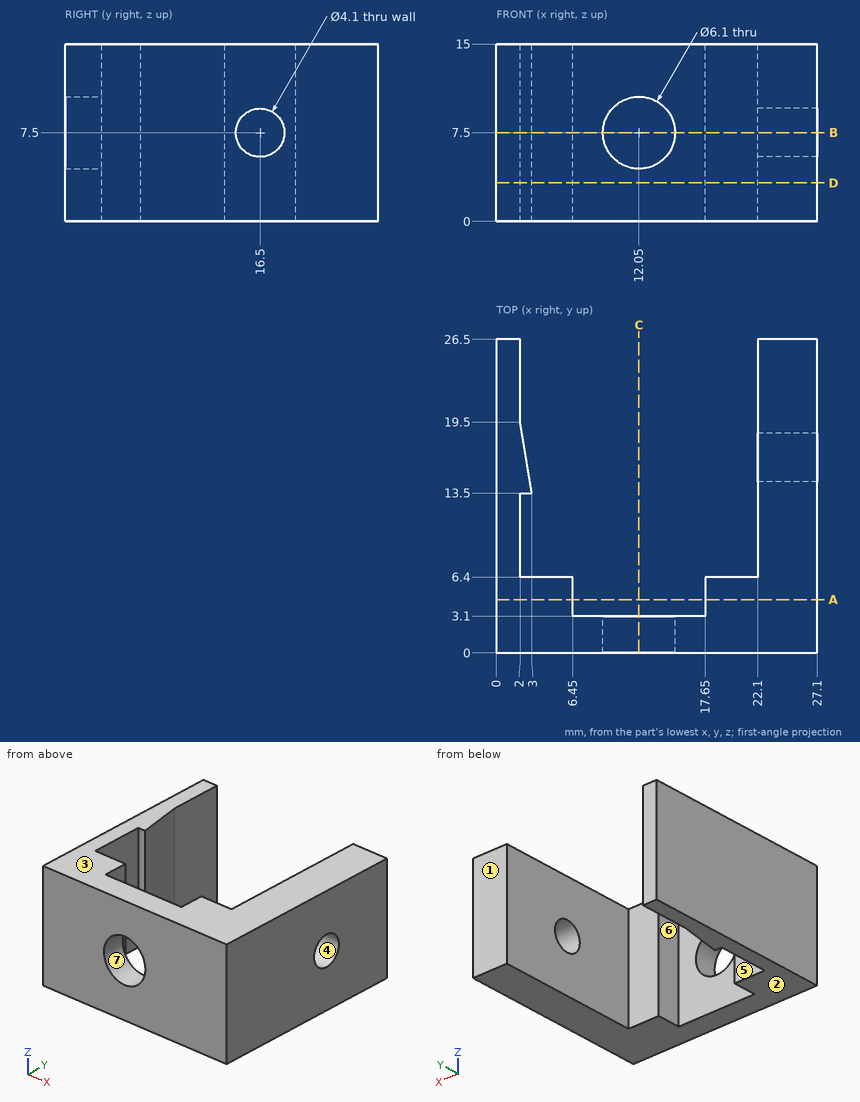
Verification items for this drawing (mm, ordinates from the low corner). A direction names the side the tool comes from. Coordinates: 2 decimals unless noted, no trailing zeros. Write each loop counter-clockwise with the first axis right and the second up, starting at its lowest first coordinate (ties: lowest second). Pieces come first, ordered by that corner, then holes. Notation, with made-up numbers: (76, 13.25) -> (100, 13.25) arc R9 cw to (100, 20.25) -> close; hole circle Ø2 at (-16.75, -34.5). An arc over 180 degrees is marked (long way). Use CSV: the item, a comma, the result in double quotes. Start each with the question number.
Item 1: Cross-section at C-C, the plane x = 12.05. Record the cut outline in (y, z).
Item 2: Thickness scan on line 1 (X direction, y = 25.25, z = 11.75); line 2 (Z direction, x = 23.1, y = 16.5); line 3 (X direction, y = 4.25, z = 9.25). Record the ranges inside material, lowest first.
Item 3: Cross-section at A-A, the plane y = 4.5. Record the cut outline in (x, z), plus the area to 4 significant figures.
Item 4: Depth check by flat-ended pin: pin 1 Ø1.3 at (x, z) = (20, 5.5) entering from +Y; pin 2 Ø1.7 at (y, z) = (5.5, 9) entering from -X; pin 3 Ø9 at (x, z) = (11, 10) entering from +Y. Enter the tip coordinate at first touch or a pass-through.
Item 5: Cross-section at D-D, the plane z = 3.25. Record the cut outline in (x, y), plus the area to 3 significant figures.
Item 6: Cross-section at B-B, the plane z = 7.5. Record the cut outline in (x, y).
Item 7: Set-up check for the marked faces 5, 6 and 7: record each of +Z, -Z, +X, -X, +Y, -Y from which the full face is reachable in a straight line by a thin tool's end or side.
Item 8: Mould release check, pull along Z, two halves, no side actions. Record for the marked faces 1, 2, 3 and 4: released by +Z, released by -Z, zero draft, split by the parting line, or undercut.
Answers:
1,outline,"(0, 0) -> (3.1, 0) -> (3.1, 4.45) -> (0, 4.45) -> close; (0, 10.55) -> (3.1, 10.55) -> (3.1, 15) -> (0, 15) -> close"
2,line 1,"0 to 2, 22.1 to 27.1"
2,line 2,"0 to 5.45, 9.55 to 15"
2,line 3,"0 to 6.45, 17.65 to 27.1"
3,outline,"(0, 0) -> (6.45, 0) -> (6.45, 15) -> (0, 15) -> close; (17.65, 0) -> (27.1, 0) -> (27.1, 15) -> (17.65, 15) -> close"
3,area,"238.5 mm^2"
4,pin 1,"y = 6.4"
4,pin 2,"x = 0"
4,pin 3,"y = 3.1"
5,outline,"(0, 0) -> (27.1, 0) -> (27.1, 26.5) -> (22.1, 26.5) -> (22.1, 6.4) -> (17.65, 6.4) -> (17.65, 3.1) -> (6.45, 3.1) -> (6.45, 6.4) -> (2, 6.4) -> (2, 13.5) -> (3, 13.5) -> (2, 19.5) -> (2, 26.5) -> (0, 26.5) -> close"
5,area,"280 mm^2"
6,outline,"(0, 0) -> (9, 0) -> (9, 3.1) -> (6.45, 3.1) -> (6.45, 6.4) -> (2, 6.4) -> (2, 13.5) -> (3, 13.5) -> (2, 19.5) -> (2, 26.5) -> (0, 26.5) -> close; (15.1, 0) -> (27.1, 0) -> (27.1, 14.45) -> (22.1, 14.45) -> (22.1, 6.4) -> (17.65, 6.4) -> (17.65, 3.1) -> (15.1, 3.1) -> close; (22.1, 18.55) -> (27.1, 18.55) -> (27.1, 26.5) -> (22.1, 26.5) -> close"
7,face 5,"+Z, -Z"
7,face 6,"+Z, -Z, +Y"
7,face 7,"+Y, -Y"
8,face 1,"zero draft"
8,face 2,"released by -Z"
8,face 3,"released by +Z"
8,face 4,"undercut"
